Check sheet for the modelled part. Datum: model origin and axes. Units: mm. A direction names the side the tool comes from. Give positions to 0.01 mm unless a question says otherwise; leave off trailing zeros. Order: outer loops, then holes, each group sorted by start corner. A loop starts at its lowest first (then second) coordinate and runs counter-clockwise, first axis right, second up.
```python
from build123d import *

# Parameters (mm, degrees)
F1_R      = 9.3853456038
F1_W      = 14.4104864448
F1_H      = 6.3965022564
F2_DEPTH  = 5.9
F4_R      = 9.0168673832
F4_W      = 14.4104864448
F4_H      = 6.3965022564
F5_DEPTH  = 13
F3_W      = 14.4104864448
F3_H      = 0.9191088029
F6_DEPTH  = 14
F8_DEPTH  = 5.5
F10_DEPTH = 13.7
F11_W     = 0.7204534382
F11_H     = 14
F12_DEPTH = 5
F13_W     = 12.9795465618
F13_H     = 0.8269683793
F14_DEPTH = 5


with BuildPart() as f2:
    # F1 (on face) → F2 (new body)
    with BuildSketch(Plane.XY):
        with Locations((-7.2333719581, -3.1627740245)):
            Circle(F1_R)
        with Locations((-7.2052432224, -3.1982511282)):
            Rectangle(F1_W, F1_H, mode=Mode.SUBTRACT)
    extrude(amount=F2_DEPTH)

    # F4 (on face) → F5 (join)
    with BuildSketch(Plane.XY):
        with Locations((-7.186296396, -3.2088013832)):
            Circle(F4_R)
        with Locations((-7.2052432224, -3.1982511282)):
            Rectangle(F4_W, F4_H, mode=Mode.SUBTRACT)
    extrude(amount=-F5_DEPTH)

    # F3 (on face) → F6 (join)
    with BuildSketch(Plane(origin=(0, 0, 0), x_dir=(1, 0, 0), z_dir=(0, 0, -1))):
        with Locations((-7.2052432224, 0.4595544015)):
            Rectangle(F3_W, F3_H)
    extrude(amount=F6_DEPTH)

    # F7 (on face) → F8 (join)
    with BuildSketch(Plane.XZ.offset(0.9191088029)):
        Polygon((-0.701982528, -14), (0, -14), (0, -13), (0, 0), (-0.701982528, 0), align=None)
    extrude(amount=F8_DEPTH)

    # F9 (on face) → F10 (join)
    with BuildSketch(Plane(origin=(-0.701982528, 0, 0), x_dir=(0, -1, 0), z_dir=(-1, 0, 0))):
        Polygon((6.3965022564, -13), (6.3965022564, 0), (5.576975178, 0), (5.576975178, -14), (6.3965022564, -14), align=None)
    extrude(amount=F10_DEPTH)

    # F11 (on face) → F12 (join)
    with BuildSketch(Plane(origin=(0, -5.576975178, 0), x_dir=(-1, 0, 0), z_dir=(0, 1, 0))):
        with Locations((14.0417558089, -7)):
            Rectangle(F11_W, F11_H)
    extrude(amount=F12_DEPTH)

    # F13 (on face) → F14 (join)
    with BuildSketch(Plane(origin=(0, -5.576975178, 0), x_dir=(-1, 0, 0), z_dir=(0, 1, 0))):
        with Locations((7.1917558089, -13.5865158103)):
            Rectangle(F13_W, F13_H)
    extrude(amount=F14_DEPTH)


solid = f2.part
```
(1) Release check for a two-part mould opening along X. For faces 1 (the face through (-7, -5.577, -6)), 2 (the face through (-14.41, -0.5, -13.5)), 3 (the face through (-7, -7, 5.9)) record: released by +X, released by -X, zero draft, split by the parting line, or undercut.
Response values:
face 1: undercut
face 2: released by -X
face 3: zero draft
(2) Set-up check for faces 4 (the face through (-7, -6, 0)), 5 (the face through (-7.3, 0, -13.5)), 6 (the face through (-7, -3, -14)), 7 (the face through (-13, 4, 0)), 8 (the face through (-7.5, -6.397, -13.5)): record each of +Z, -Z, +X, -X, +Y, -Y from which the full face is reachable in a straight line by a thin tool's end or side.
Response values:
face 4: +Z
face 5: -Z, +X, -X, +Y
face 6: -Z, +X, -X, +Y, -Y
face 7: -Z
face 8: -Z, -X, -Y
(3) Cross-section at C-C on x = -2.5. Enter the section's corners in (y, z).
Response values:
outline: (-11.27, 0) - (-10.91, 0) - (-10.91, -13) - (-6.4, -13) - (-6.4, -14) - (0, -14) - (0, -13) - (4.49, -13) - (4.49, 0) - (4.94, 0) - (4.94, 5.9) - (0, 5.9) - (0, 0) - (-0.92, 0) - (-0.92, -13.17) - (-5.58, -13.17) - (-5.58, 0) - (-6.4, 0) - (-6.4, 5.9) - (-11.27, 5.9) - close
(4) Cross-section at A-A on y = -6. Enter the section's corners in (x, z), then the cut area to 3 significant figures.
Response values:
outline: (-16.18, 0) - (-15.76, 0) - (-15.76, -13) - (-14.41, -13) - (-14.41, 5.9) - (-16.18, 5.9) - close; (-14.4, -14) - (0, -14) - (0, -13) - (1.39, -13) - (1.39, 0) - (1.71, 0) - (1.71, 5.9) - (0, 5.9) - (0, 0) - (-14.4, 0) - close
area: 258 mm2
(5) Cross-section at D-D on y = -10.5. Enter the section's corners in (x, z).
Response values:
outline: (-13.09, 0) - (-12.49, 0) - (-12.49, -13) - (-1.88, -13) - (-1.88, 0) - (-1.38, 0) - (-1.38, 5.9) - (-13.09, 5.9) - close
(6) Cross-section at B-B on z = -8.5. Count the separate pieces of the cut face and the enclosed holes in it, then the cut area to 3 significant figures.
Response values:
separate pieces: 1
enclosed holes: 2
area: 195 mm2
(7) Gauge pin test, flat ends, axial feed: pin 1 Ø8 at (x, z) = (-9, -10) entering from +Y; pin 2 Ø1.1 at (y, z) = (-2, -13.5) entering from +X; pin 3 Ø4.5 at (y, z) = (-5, -6) entering from -X. Record the tip position at first contact, or that the pin passes through.
Response values:
pin 1: stops at y = 5.81
pin 2: stops at x = 1.78
pin 3: stops at x = -16.2
(8) Material ranges on L1, parallel to Z at x = -6.25, y = -4.25; L2, parallel to Z at x = -6, y = 1; L3, parallel to Y at x = -8.5, z = -3, recorded low to high.
Response values:
L1: z = -14 to -13.17
L2: z = -13 to 5.9
L3: y = -12.13 to -5.58, -0.92 to 5.71
